Geometry check sheet. Reference: the model listing, model coordinates, mm. Coordinates: 2 decimals unless noted, no trailing zeros. Order: outer loops, then holes, each group sorted by start corner. A loop starts at its lowest first (then second) coordinate and runs counter-clockwise, first axis right, second up. Notation, with made-up numbers: (20.25, 45) - (65.25, 45) arc R22 ccw to (65.25, 53) - close; hole circle Ø10 at (36.5, 71.25). An arc over 180 degrees is marked (long way). Use CSV: the item, a comma, the result in double quotes. Start each with the question number.
1) Thickness scan on probe 1 along X at (y, z) = (5, 4.15); probe 2 along Z at (x, y) = (15, 5.75); probe 3 along X at (y, z) = (7.25, 1.2). Record the ranges inside material, lowest first. Write a range as [from, to].
2) Depth check by flat-ended pin: P1, Ø2, axis at x = 10, y = 4.5, coming from the -Z side. Enter the tip coordinate at first touch or a pass-through.
3) Sectioned sample at C-C, the plane z = 0.5. Record the cut outline in (x, y).
4) Sectioned sample at A-A, the plane x = 4. Record the cut outline in (y, z).
5) Sectioned sample at D-D, the plane x = 7.5. Record the cut outline in (y, z), and give its area (3 significant figures).
6) Sectioned sample at B-B, the plane y = 5.5. Record the cut outline in (x, z), and give its area (3 significant figures).
from build123d import *

# Parameters (mm, degrees)
SKETCH003_R      = 2.5
EXTRUDE003_DEPTH = 1
CHAMFER_SIZE     = 0.1
SKETCH006_W      = 20
SKETCH006_H      = 7
EXTRUDE018_DEPTH = 0.5
SKETCH001_W      = 1
SKETCH001_H      = 3
EXTRUDE001_DEPTH = 1
SKETCH002_W      = 1
SKETCH002_H      = 3
EXTRUDE002_DEPTH = 1
SKETCH_W         = 22
SKETCH_H         = 9
EXTRUDE_DEPTH    = 3
CHAMFER001_SIZE  = 0.5


with BuildPart() as chamfer001:
    # Sketch003 → Extrude003 (new body)
    with BuildSketch(Plane(origin=(-0.5, 0, 0), x_dir=(1, 0, 0), z_dir=(0, 0, 1))):
        with Locations((6.5, 5.5)):
            Circle(SKETCH003_R)
    extrude(amount=EXTRUDE003_DEPTH)

    # Chamfer
    chamfer_edges = [chamfer001.edges().sort_by_distance(p)[0] for p in [
        (3.5, 5.5, 0),
    ]]
    chamfer(chamfer_edges, length=CHAMFER_SIZE)


with BuildPart() as chamfer001_1:
    # Chamfer placement: moved
    add(chamfer001.part.moved(Location((-2, 0, 0))))


with BuildPart() as fusion020:
    # Sketch006 → Extrude018 (new body)
    with BuildSketch(Plane.XY.offset(1)):
        with Locations((9, 5.5)):
            Rectangle(SKETCH006_W, SKETCH006_H)
    extrude(amount=EXTRUDE018_DEPTH)

    # Fusion020: union Chamfer001
    add(chamfer001_1.part)


with BuildPart() as extrude001:
    # Sketch001 → Extrude001 (new body)
    with BuildSketch(Plane(origin=(0, 1, 4), x_dir=(1, 0, 0), z_dir=(0, 0, 1))):
        with Locations((0.75, 4.5)):
            Rectangle(SKETCH001_W, SKETCH001_H)
    extrude(amount=EXTRUDE001_DEPTH)


with BuildPart() as extrude001_1:
    # Extrude001 placement: moved
    add(extrude001.part.moved(Location((-2, 0, 0))))


with BuildPart() as fusion:
    # Sketch002 → Extrude002 (new body)
    with BuildSketch(Plane(origin=(18.5, 1, 4), x_dir=(1, 0, 0), z_dir=(0, 0, 1))):
        with Locations((0.75, 4.5)):
            Rectangle(SKETCH002_W, SKETCH002_H)
    extrude(amount=EXTRUDE002_DEPTH)

    # Fusion: union Extrude001
    add(extrude001_1.part)


with BuildPart() as body:
    # Sketch → Extrude (new body)
    with BuildSketch(Plane.XY.offset(1.5)):
        with Locations((9, 5.5)):
            Rectangle(SKETCH_W, SKETCH_H)
    extrude(amount=EXTRUDE_DEPTH)

    # Chamfer001
    chamfer001_edges = [body.edges().sort_by_distance(p)[0] for p in [
        (20, 5.5, 1.5),
        (-2, 5.5, 1.5),
    ]]
    chamfer(chamfer001_edges, length=CHAMFER001_SIZE)

    # Cut: cut Fusion
    add(fusion.part, mode=Mode.SUBTRACT)

    # Fusion021: union Fusion020
    add(fusion020.part)


solid = body.part
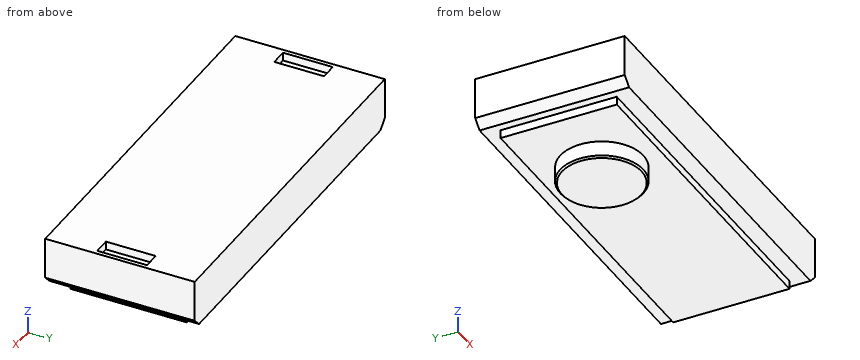
Evaluation:
1,probe 1,"[-2, -1.75], [-0.75, 18.75], [19.75, 20]"
1,probe 2,"[1, 4.5]"
1,probe 3,"[-1, 19]"
2,P1,"z = 1"
3,outline,"circle Ø5 at (4, 5.5)"
4,outline,"(1, 1.5) - (2, 1.5) - (2, 1) - (3, 1) - (3, 0.1) - (3.1, 0) - (7.9, 0) - (8, 0.1) - (8, 1) - (9, 1) - (9, 1.5) - (10, 1.5) - (10, 4.5) - (1, 4.5) - close"
5,outline,"(1, 1.5) - (2, 1.5) - (2, 1) - (9, 1) - (9, 1.5) - (10, 1.5) - (10, 4.5) - (1, 4.5) - close"
5,area,"30.5 mm²"
6,outline,"(-2, 2) - (-1.5, 1.5) - (-1, 1.5) - (-1, 1) - (1.5, 1) - (1.5, 0.1) - (1.6, 0) - (6.4, 0) - (6.5, 0.1) - (6.5, 1) - (19, 1) - (19, 1.5) - (19.5, 1.5) - (20, 2) - (20, 4.5) - (19.75, 4.5) - (19.75, 4) - (18.75, 4) - (18.75, 4.5) - (-0.75, 4.5) - (-0.75, 4) - (-1.75, 4) - (-1.75, 4.5) - (-2, 4.5) - close"
6,area,"79.7 mm²"
